Design review of the part built by this model. Coordinates are the model's own, in mm. Face numbers are marked on the shaded views. A direction names the side the tool comes from. Give positions to 0.01 mm unless a question says otherwise; leave off trailing zeros. Write each loop counter-clockwise with the first axis right and the second up, starting at its lowest first coordinate (ties: lowest second). Pieces come first, ordered by that corner, then holes.
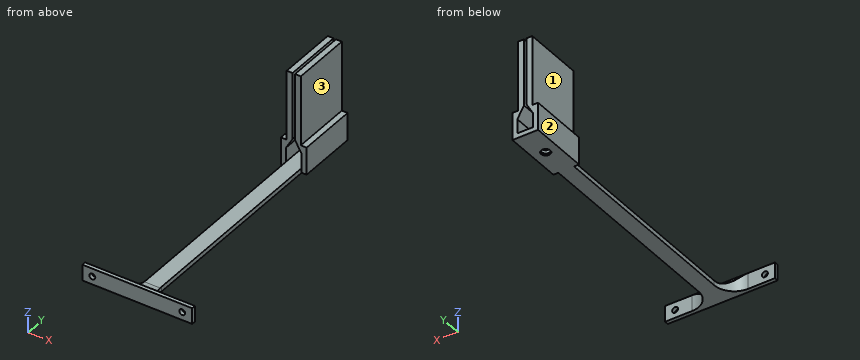
```python
from build123d import *
from build123d.topology import SkipClean

# Parameters (mm, degrees)
SKETCH1_W           = 10
SKETCH1_H           = 170.55
SKETCH1_R           = 2.5
BOSS_EXTRUDE1_DEPTH = 2
SKETCH2_W           = 10
SKETCH2_H           = 170.55
SKETCH2_R           = 2.95
BOSS_EXTRUDE2_DEPTH = 1
SKETCH3_W           = 69.85
SKETCH3_H           = 10.16
SKETCH3_R           = 1.86055
BOSS_EXTRUDE3_DEPTH = 2.5
FILLET1_START       = -1
FILLET1_DEPTH       = 10.16
FILLET1_START_2     = -17.7000001
FILLET1_2_DEPTH     = 35.4000001
FILLET1_START_3     = -5
FILLET1_3_DEPTH     = 10
SKETCH4_W           = 10
SKETCH4_H           = 13.05
BOSS_EXTRUDE4_DEPTH = 3
SKETCH4_3_W         = 3.175
SKETCH4_3_H         = 38.1
BOSS_EXTRUDE5_DEPTH = 11.1125
SKETCH5_W           = 7.38125
SKETCH5_H           = 38.1
BOSS_EXTRUDE6_DEPTH = 50.8
SKETCH6_W           = 3.690625
SKETCH6_H           = 38.1
CUT_EXTRUDE1_DEPTH  = 44.45
CHAMFER1_SIZE       = 4.7625
CHAMFER1_SIZE_2     = 8.248891971


with BuildPart() as part:
    # Sketch1 → Boss-Extrude1 (new body)
    with BuildSketch(Plane.XY):
        with Locations((0, 3)):
            Rectangle(SKETCH1_W, SKETCH1_H)
        with Locations((0, 82.275)):
            Circle(SKETCH1_R, mode=Mode.SUBTRACT)
    extrude(amount=BOSS_EXTRUDE1_DEPTH)

    # Sketch2 → Boss-Extrude2 (add)
    with BuildSketch(Plane(origin=(0, 0, 0), x_dir=(-1, 0, 0), z_dir=(0, 0, -1))):
        with Locations((0, 3)):
            Rectangle(SKETCH2_W, SKETCH2_H)
        with Locations((0, 82.275)):
            Circle(SKETCH2_R, mode=Mode.SUBTRACT)
    extrude(amount=BOSS_EXTRUDE2_DEPTH)

    # Sketch3 → Boss-Extrude3 (add)
    with BuildSketch(Plane.XZ.offset(82.275)):
        with Locations((0, 4.08)):
            Rectangle(SKETCH3_W, SKETCH3_H)
        with Locations(Location((28.575, 4.08, 0), (0, 0, 270))):
            Circle(SKETCH3_R, mode=Mode.SUBTRACT)
        with Locations(Location((-28.575, 4.08, 0), (0, 0, 270))):
            Circle(SKETCH3_R, mode=Mode.SUBTRACT)
    extrude(amount=-BOSS_EXTRUDE3_DEPTH)

    # Fillet1: read off the stored shape, not the designer's step
    # Fillet1 outline → Fillet1 (add)
    with BuildSketch(Plane.XY.offset(FILLET1_START)):
        with BuildLine():
            Line((5, -79.775), (17.7, -79.775))
            ThreePointArc((17.7, -79.775), (8.719743879, -76.055256121), (5, -67.075))
            Line((5, -67.075), (5, -79.775))
        make_face()
        with BuildLine():
            Line((-17.7, -79.775), (-5, -79.775))
            Line((-5, -79.775), (-5, -67.075))
            ThreePointArc((-5, -67.075), (-8.719743879, -76.055256121), (-17.7, -79.775))
        make_face()
    extrude(amount=FILLET1_DEPTH)

    # Fillet1 2 outline → Fillet1 2 (cut)
    with BuildSketch(Plane.YZ.offset(FILLET1_START_2)):
        with BuildLine():
            Line((-66, 9.16), (-79.775009155, 9.160018885))
            ThreePointArc((-79.775009155, 9.160018885), (-75.089891257, 3.937849653), (-68.347034302, 2))
            Line((-68.347034302, 2), (-66, 2))
            Line((-66, 2), (-66, 9.16))
        make_face()
    extrude(amount=FILLET1_2_DEPTH, mode=Mode.SUBTRACT)

    # Fillet1 3 outline → Fillet1 3 (add)
    with SkipClean():  # the faces are left unmerged after this step: merging them gives an invalid solid
        with BuildSketch(Plane.YZ.offset(FILLET1_START_3)):
            with BuildLine():
                ThreePointArc((-68.347034302, 2), (-75.089891257, 3.937849653), (-79.775009155, 9.160018885))
                Line((-79.775009155, 9.160018885), (-79.775, 0))
                Line((-79.775, 0), (-66, 0))
                Line((-66, 0), (-66, 2))
                Line((-66, 2), (-68.347034302, 2))
            make_face()
        extrude(amount=FILLET1_3_DEPTH)
    add(part.part.scale(1), mode=Mode.REPLACE)  # the faces are merged on a copy

    # Sketch4 → Boss-Extrude4 (add)
    with SkipClean():  # the faces are left unmerged after this step: merging them gives an invalid solid
        with BuildSketch(Plane(origin=(0, 0, -1), x_dir=(-1, 0, 0), z_dir=(0, 0, -1))):
            Polygon((8.175, 63.225), (8.175, 101.325), (5, 101.325), (5, 88.275), (5, 63.225), align=None)
            with Locations((0, 94.8)):
                Rectangle(SKETCH4_W, SKETCH4_H)
            Polygon((-5, 88.275), (-5, 101.325), (-8.175, 101.325), (-8.175, 63.225), (-5, 63.225), align=None)
        extrude(amount=-BOSS_EXTRUDE4_DEPTH)

    # Sketch4<3> → Boss-Extrude5 (add)
    with SkipClean():  # the faces are left unmerged after this step: merging them gives an invalid solid
        with BuildSketch(Plane(origin=(0, 0, -1), x_dir=(-1, 0, 0), z_dir=(0, 0, -1))):
            with Locations((6.5875, 82.275)):
                Rectangle(SKETCH4_3_W, SKETCH4_3_H)
            with Locations((-6.5875, 82.275)):
                Rectangle(SKETCH4_3_W, SKETCH4_3_H)
        extrude(amount=-BOSS_EXTRUDE5_DEPTH)

    # Sketch5 → Boss-Extrude6 (add)
    with SkipClean():  # the faces are left unmerged after this step: merging them gives an invalid solid
        with BuildSketch(Plane.XY.offset(10.1125)):
            with Locations((-4.484375, 82.275)):
                Rectangle(SKETCH5_W, SKETCH5_H)
            with Locations((4.484375, 82.275)):
                Rectangle(SKETCH5_W, SKETCH5_H)
        extrude(amount=BOSS_EXTRUDE6_DEPTH)

    # Sketch6 → Cut-Extrude1 (cut)
    with SkipClean():  # the faces are left unmerged after this step: merging them gives an invalid solid
        with BuildSketch(Plane.XY.offset(60.9125)):
            with Locations((-6.3296875, 82.275)):
                Rectangle(SKETCH6_W, SKETCH6_H)
            with Locations((6.3296875, 82.275)):
                Rectangle(SKETCH6_W, SKETCH6_H)
        extrude(amount=-CUT_EXTRUDE1_DEPTH, mode=Mode.SUBTRACT)

    # Chamfer1
    # the kernel refuses this chamfer: 8.248891971, 4.7625 mm, written as the material it takes off along each edge
    with BuildSketch(Plane(origin=(-0.79375, 122.66559091, 10.1125), x_dir=(-1, 0, 0), z_dir=(0, -1, 0))) as chamfer1_piece_1_section:
        Polygon((CHAMFER1_SIZE, 0), (0, -CHAMFER1_SIZE_2), (0, 0), align=None)
    chamfer1_piece_1 = extrude(amount=80.78118182, mode=Mode.PRIVATE)
    chamfer1_piece_1 = split(chamfer1_piece_1, bisect_by=Plane(origin=(-5, 122.66559091, 10.1125), z_dir=(1, 0, 0)), keep=Keep.TOP, mode=Mode.PRIVATE)
    add(chamfer1_piece_1, mode=Mode.SUBTRACT)
    with BuildSketch(Plane(origin=(0.79375, 122.66559091, 10.1125), x_dir=(1, 0, 0), z_dir=(0, -1, 0))) as chamfer1_piece_2_section:
        Polygon((CHAMFER1_SIZE, 0), (0, CHAMFER1_SIZE_2), (0, 0), align=None)
    chamfer1_piece_2 = extrude(amount=80.78118182, mode=Mode.PRIVATE)
    chamfer1_piece_2 = split(chamfer1_piece_2, bisect_by=Plane(origin=(5, 122.66559091, 10.1125), z_dir=(-1, 0, 0)), keep=Keep.TOP, mode=Mode.PRIVATE)
    add(chamfer1_piece_2, mode=Mode.SUBTRACT)


solid = part.part
```
(1) Consider section D-D, the plane y = -59. Give the boundary of the cut face in (x, z).
Resolved:
outline: (-5, -1) - (5, -1) - (5, 2) - (-5, 2) - close
(2) Consider section C-C, the plane x = -10. Give the boundary of the cut face in (y, z) (1 decimal).
Resolved:
outline: (-82.3, -1) - (-77.2, -1) - (-77.2, 5.6) arc R12.7 cw to (-79.8, 9.2) - (-82.3, 9.2) - close
(3) To check wall thickness, follow L1, parallel to X at y = -81.3, z = 4.08 (3 decimals); L2, parallel to X at y = 91.5, z = 33.5; L3, parallel to Y at x = 0, z = -0.2 (3 decimals). State the ranges of each line that lie inside material, in increasing order.
Resolved:
L1: x = -34.925 to -30.436, -26.714 to 26.714, 30.436 to 34.925
L2: x = -4.48 to -0.79, 0.79 to 4.48
L3: y = -82.275 to 79.325, 85.225 to 101.325
(4) Consider section B-B, the plane z = 4.08. Give the boundary of the cut face in (x, y) (3 decimals).
Resolved:
outline: (-34.925, -82.275) - (-30.436, -82.275) - (-30.436, -79.775) - (-34.925, -79.775) - close; (-26.714, -82.275) - (26.714, -82.275) - (26.714, -79.775) - (17.7, -79.775) arc R12.7 cw to (8.033, -75.312) - (-8.033, -75.312) arc R12.7 cw to (-17.7, -79.775) - (-26.714, -79.775) - close; (-8.175, 63.225) - (-5, 63.225) - (-5, 101.325) - (-8.175, 101.325) - close; (5, 63.225) - (8.175, 63.225) - (8.175, 101.325) - (5, 101.325) - close; (30.436, -82.275) - (34.925, -82.275) - (34.925, -79.775) - (30.436, -79.775) - close
(5) Tool access review of the marked faces 1, 2 and 3: name each direction out of +Z, -Z, +X, -X, +Y, -Y from which nothing blocks a thin tool from reaching the whole face with its end or side.
Resolved:
face 1: +Z, -X, +Y, -Y
face 2: +Z, -Z, -X, +Y
face 3: +Z, +X, +Y, -Y
(6) Clearance check with flat-ended pins moving along their axes: P1, Ø4.5, axis at x = -28.575, z = 4.08, coming from the +Y side (3 decimals); P2, Ø19, axis at y = 85, z = 8, coming from the -X side (3 decimals); P3, Ø2.5, axis at y = 12, z = 0, coming from the +X side. State where each tip first meets the part, or that it passes through.
Resolved:
P1: stops at y = -79.775
P2: stops at x = -8.175
P3: stops at x = 5
(7) Consider section A-A, the plane z = 54. Give the boundary of the cut face in (x, y) (3 decimals), then the cut area to 3 significant figures.
Resolved:
outline: (-4.484, 63.225) - (-0.794, 63.225) - (-0.794, 101.325) - (-4.484, 101.325) - close; (0.794, 63.225) - (4.484, 63.225) - (4.484, 101.325) - (0.794, 101.325) - close
area: 281 mm2
